from build123d import *

# Parameters (mm, degrees)
BOSS_EXTRUDE1_DEPTH = 2


with BuildPart() as part:
    # Sketch4 → Boss-Extrude1 (new body)
    with BuildSketch(Plane(origin=(0, 0, 0), x_dir=(0, 0, -1), z_dir=(1, 0, 0))):
        with BuildLine():
            Line((34.101087746, -13.088045862), (34.101087746, -4.462231487))
            ThreePointArc((34.101087746, -4.462231487), (33.899842921, -3.9763835), (33.413994934, -3.775138674))
            Line((33.413994934, -3.775138674), (31.351087746, -3.775138674))
            Line((31.351087746, -3.775138674), (31.351087746, -5.775138674))
            ThreePointArc((31.351087746, -5.775138674), (30.851087746, -6.275138674), (30.351087746, -5.775138674))
            Line((30.351087746, -5.775138674), (26.851087746, -5.775138674))
            ThreePointArc((26.851087746, -5.775138674), (26.351087746, -6.275138674), (25.851087746, -5.775138674))
            Line((25.851087746, -5.775138674), (25.851087746, -3.775138674))
            Line((25.851087746, -3.775138674), (21.233669279, -3.775138674))
            Line((21.233669279, -3.775138674), (12.233669279, -5.275138674))
            Line((12.233669279, -5.275138674), (-8.644965801, -5.275138674))
            ThreePointArc((-8.644965801, -5.275138674), (-14.710069272, -3.705121285), (-19.251601877, 0.610538145))
            Line((-19.251601877, 0.610538145), (-30.235935202, 18.224861326))
            Line((-30.235935202, 18.224861326), (-31.434679787, 18.224861326))
            ThreePointArc((-31.434679787, 18.224861326), (-31.839000225, 17.820540888), (-32.243320663, 18.224861326))
            Line((-32.243320663, 18.224861326), (-32.243320663, 19.724861326))
            ThreePointArc((-32.243320663, 19.724861326), (-32.389767272, 20.078414716), (-32.743320663, 20.224861326))
            Line((-32.743320663, 20.224861326), (-37.743320663, 20.224861326))
            ThreePointArc((-37.743320663, 20.224861326), (-38.096874053, 20.078414716), (-38.243320663, 19.724861326))
            Line((-38.243320663, 19.724861326), (-38.243320663, 18.224861326))
            ThreePointArc((-38.243320663, 18.224861326), (-38.647641101, 17.820540888), (-39.051961539, 18.224861326))
            Line((-39.051961539, 18.224861326), (-40.090546725, 18.224861326))
            Line((-40.090546725, 18.224861326), (-40.090546725, 15.063013808))
            ThreePointArc((-40.090546725, 15.063013808), (-39.78872162, 13.538709885), (-38.928795501, 12.244442559))
            ThreePointArc((-38.928795501, 12.244442559), (-36.430620964, 9.401503447), (-34.296876278, 6.275753549))
            ThreePointArc((-34.296876278, 6.275753549), (-32.973480494, -3.425461249), (-39.047864509, -11.104445805))
            ThreePointArc((-39.047864509, -11.104445805), (-39.810232099, -11.839329581), (-40.090546725, -12.860447701))
            Line((-40.090546725, -12.860447701), (-40.090546725, -13.775138674))
            Line((-40.090546725, -13.775138674), (-39.051961539, -13.775138674))
            ThreePointArc((-39.051961539, -13.775138674), (-38.647641101, -13.370818236), (-38.243320663, -13.775138674))
            Line((-38.243320663, -13.775138674), (-38.243320663, -15.275138674))
            ThreePointArc((-38.243320663, -15.275138674), (-38.096874053, -15.628692065), (-37.743320663, -15.775138674))
            Line((-37.743320663, -15.775138674), (-32.743320663, -15.775138674))
            ThreePointArc((-32.743320663, -15.775138674), (-32.389767272, -15.628692065), (-32.243320663, -15.275138674))
            Line((-32.243320663, -15.275138674), (-32.243320663, -13.775138674))
            ThreePointArc((-32.243320663, -13.775138674), (-31.839000225, -13.370818236), (-31.434679787, -13.775138674))
            Line((-31.434679787, -13.775138674), (22.101087746, -13.775138674))
            ThreePointArc((22.101087746, -13.775138674), (22.601087746, -13.275138674), (23.101087746, -13.775138674))
            Line((23.101087746, -13.775138674), (23.101087746, -15.275138674))
            ThreePointArc((23.101087746, -15.275138674), (23.247534356, -15.628692065), (23.601087746, -15.775138674))
            Line((23.601087746, -15.775138674), (28.601087746, -15.775138674))
            ThreePointArc((28.601087746, -15.775138674), (28.954641137, -15.628692065), (29.101087746, -15.275138674))
            Line((29.101087746, -15.275138674), (29.101087746, -13.775138674))
            ThreePointArc((29.101087746, -13.775138674), (29.601087746, -13.275138674), (30.101087746, -13.775138674))
            Line((30.101087746, -13.775138674), (33.413994934, -13.775138674))
            ThreePointArc((33.413994934, -13.775138674), (33.899842921, -13.573893849), (34.101087746, -13.088045862))
        make_face()
    extrude(amount=BOSS_EXTRUDE1_DEPTH)


solid = part.part
CAD build for the part. Positions are in the model's coordinates, mm. A direction names the side the tool comes from. Round coordinates to 2 decimals unless told otherwise and drop trailing zeros. Loops run counter-clockwise (first coordinate to the right, second up) from the corner with the lowest first, then second, coordinate; pieces in that order, holes last. Notation, with made-up numbers: (-3, 74) - (39, 74) arc R23 ccw to (39, 92) - close; hole circle Ø7 at (-31.75, -31.75). An arc over 180 degrees is marked (long way). Put each result on its own line as item: value.
1. Two-plate mould, pull along Z, no slides. Class faces 5 (the flat face through (2, -6, 12)), 6 (the cylindrical face through (0.986, -3.289, 32.937)), 7 (the flat face through (1, -15, -23.101)): released by +Z, released by -Z, zero draft, split by the parting line, or undercut.
Geometry check:
face 5: zero draft
face 6: released by +Z
face 7: undercut
2. Slice it at A-A on z = -2. List the corners of the cut face in (x, y), and give its area (3 significant figures).
Geometry check:
outline: (0, -13.78) - (2, -13.78) - (2, -5.28) - (0, -5.28) - close
area: 17.0 mm²
3. Slice it at B-B on y = -8. List the corners of the cut face in (x, z), and give its area (3 significant figures).
Geometry check:
outline: (0, -34.1) - (2, -34.1) - (2, 35.32) - (0, 35.32) - close
area: 139 mm²
4. 3-axis set-ups, long thin cutter, end or side, ignore diameter. For faces 1 (the flat face through (1, -5, -31.351)), 2 (the flat face through (1, -13.775, 5)), 3 (the flat face through (1, -15, -29.101)), 4 (the flat face through (1, -15, 38.243)): which of +Z, -Z, +X, -X, +Y, -Y reach the whole face in a straight line?
Geometry check:
face 1: +X, -X, +Y
face 2: +X, -X, -Y
face 3: -Z, +X, -X, -Y
face 4: +Z, +X, -X, -Y
5. Wall check: line 1 (Y direction, x = 1.1, z = 5.5); line 2 (Y direction, x = 1.6, z = 37); line 3 (Y direction, x = 0.4, z = -28.5). Give the ranges that are in metal, low to high.
Geometry check:
line 1: -13.78 to -5.28
line 2: -15.78 to -9.71, 10.11 to 20.22
line 3: -15.78 to -5.78
6. Pin check, flat tips, straight feed: P1, Ø4, axis at y = -3.5, z = -23.5, coming from the -X side; P2, Ø0.8, axis at x = 1, y = -14.5, coming from the +Z side; P3, Ø1.2, axis at x = 1, y = -14.5, coming from the -Z side; P4, Ø1, axis at x = 1, z = -32, coming from the +Y side. Stop position of each tip, or through.
Geometry check:
P1: x = 0
P2: z = 38.24
P3: z = -29.1
P4: y = -3.78
